Check sheet for the drawn part. Datum: minimum x, y, z corner. Units: mm. A direction names the side the tool comes from. Give positions to 0.01 mm unless a question says otherwise; leave off trailing zeros. Order: outer loops, then holes, each group sorted by start corner. A loop starts at its lowest first (then second) coordinate and runs counter-clockwise, first axis right, second up. Notation, with made-up numbers: (-18.75, 12.5) - (30.25, 12.5) arc R29 ccw to (30.25, 32.5) - close; hole circle Ø5 at (-16.5, -23). An arc over 180 degrees is marked (long way). Answer as a JSON object with one key per item and string values. Group by question number.
(1) Mould release check, pull along X, two halves, no side actions. Record for the marked faces 1, 2 and 3: +X half, -X half, draft (parallel to the pull), parting line (faces both ways), or undercut.
(2) Section check B-B (z = 5). Record the boundary of the cut face in (x, y).
(3) Thickness scan on line 1 (X direction, y = 29.5, z = 3); line 2 (X direction, y = 10.5, z = 5); line 3 (Y direction, x = 12.4, z = 5). Record the ranges inside material, lowest first.
(4) Depth check by flat-ended pin: pin 1 Ø1 at (y, z) = (19, 12.5) entering from +X; pin 2 Ø0.6 at (x, y) = (8.5, 25.5) entering from +Z; pin 3 Ø1.6 at (x, z) = (8.5, 5.5) entering from +Y. Enter the tip coordinate at first touch or a pass-through.
(5) Section check A-A (y = 26.5). Record the boundary of the cut face in (x, z).
(6) Section check C-C (z = 8). Record the boundary of the cut face in (x, y).
(7) Access from +Z, -Z, +X, -X, +Y, -Y to the whole of each face (thin tool, end or side, straight path). Record for the marked faces 4, 5, 6 and 7.
(8) Section check D-D (y = 10.5). Record the boundary of the cut face in (x, z).
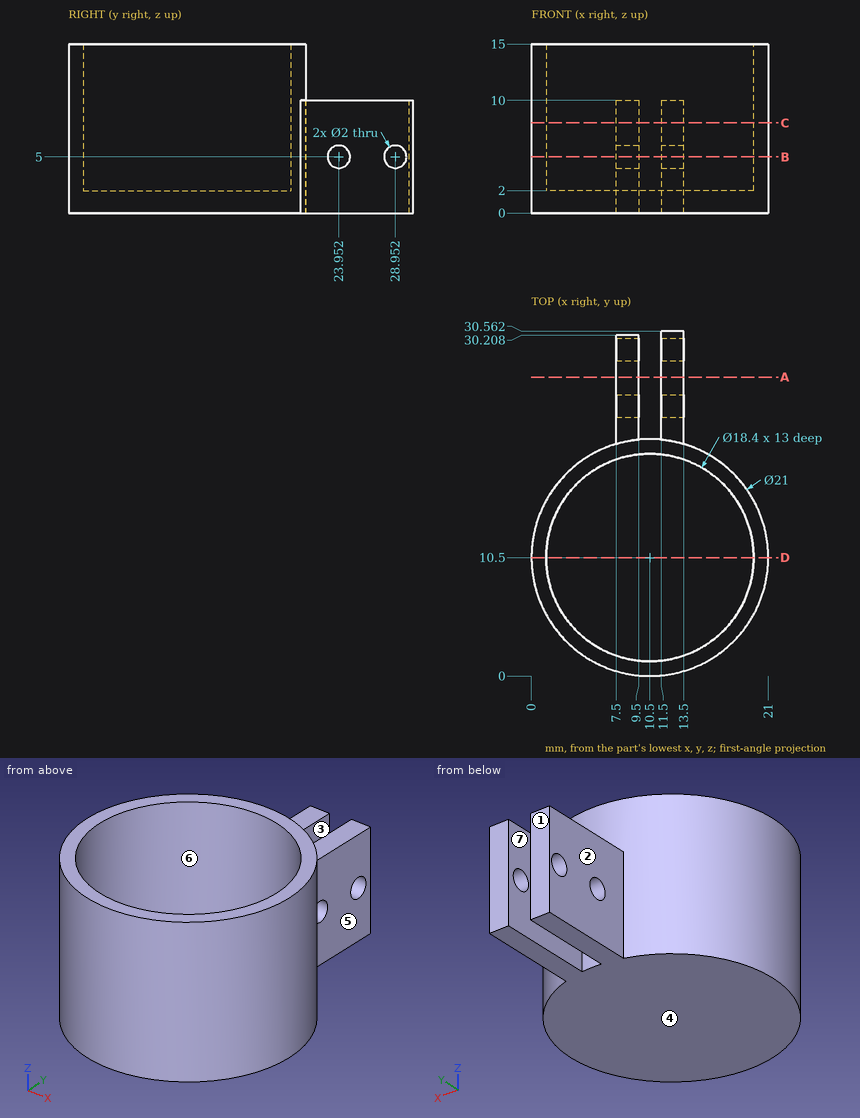
Solutions:
{
 "1": {"face 1": "draft", "face 2": "-X half", "face 3": "undercut"},
 "2": {"outline": "(7.5, 20.56) arc R10.5 ccw (long way) to (13.5, 20.56) - (13.5, 22.95) - (11.5, 22.95) - (11.5, 20.95) arc R10.5 ccw to (9.5, 20.95) - (9.5, 22.95) - (7.5, 22.95) - close; (7.5, 24.95) - (9.5, 24.95) - (9.5, 27.95) - (7.5, 27.95) - close; (7.5, 29.95) - (9.5, 29.95) - (9.5, 30.21) - (7.5, 30.21) - close; (11.5, 24.95) - (13.5, 24.95) - (13.5, 27.95) - (11.5, 27.95) - close; (11.5, 29.95) - (13.5, 29.95) - (13.5, 30.56) - (11.5, 30.56) - close; hole circle Ø18.4 at (10.5, 10.5)"},
 "3": {"line 1": "x = 7.5 to 9.5, 11.5 to 13.5", "line 2": "x = 0 to 1.3, 19.7 to 21", "line 3": "y = 0.17 to 1.5, 19.5 to 22.95, 24.95 to 27.95, 29.95 to 30.56"},
 "4": {"pin 1": "stops at x = 17.3", "pin 2": "stops at z = 10", "pin 3": "stops at y = 30.21"},
 "5": {"outline": "(7.5, 0) - (9.5, 0) - (9.5, 10) - (7.5, 10) - close; (11.5, 0) - (13.5, 0) - (13.5, 10) - (11.5, 10) - close"},
 "6": {"outline": "(7.5, 20.56) arc R10.5 ccw (long way) to (13.5, 20.56) - (13.5, 30.56) - (11.5, 30.56) - (11.5, 20.95) arc R10.5 ccw to (9.5, 20.95) - (9.5, 30.21) - (7.5, 30.21) - close; hole circle Ø18.4 at (10.5, 10.5)"},
 "7": {"face 4": "-Z, +X, -X, +Y, -Y", "face 5": "+Z, -Z, +X, +Y", "face 6": "+Z", "face 7": "+Z, -Z, +Y"},
 "8": {"outline": "(0, 0) - (21, 0) - (21, 15) - (19.7, 15) - (19.7, 2) - (1.3, 2) - (1.3, 15) - (0, 15) - close"}
}
